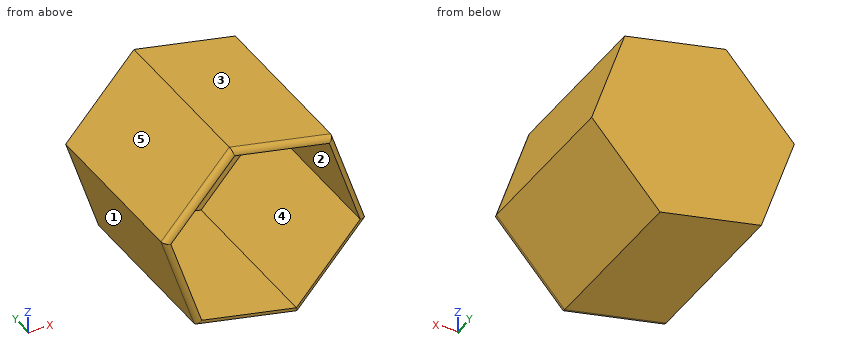
```python
from build123d import *

# Parameters (mm, degrees)
F1_DEPTH = 30
F2_T     = -1
F3_R     = 0.99999


# Not quite as in the source:
# - a fillet or chamfer is up to 0.001 mm smaller than in the source, because OpenCascade refuses the exact size


with BuildPart() as f1:
    # F0 (on Front) → F1 (new body)
    with BuildSketch(Plane.XZ):
        Polygon((-16.0683598468, 10.3036999003), (-4.4305566599, 23.5195108458), (-10.0568830769, 40.2060495226), (-27.3210126808, 43.676777254), (-38.9588158677, 30.4609663085), (-33.3324894507, 13.7744276316), align=None)
    extrude(amount=F1_DEPTH)

    # F2
    f2_openings = [f1.faces().sort_by_distance(p)[0] for p in [
        (-21.694686, -30, 26.990239),
    ]]
    offset(amount=F2_T, openings=f2_openings)

    # F3 (radius 1 in the source; OpenCascade refuses exactly that, so slightly less here)
    f3_edges = [f1.edges().sort_by_distance(p)[0] for p in [
        (-18.688948, -30, 41.941413),
        (-7.24372, -30, 31.86278),
        (-10.249458, -30, 16.911605),
        (-24.700425, -30, 12.039064),
        (-36.145653, -30, 22.117697),
        (-33.139914, -30, 37.068872),
    ]]
    fillet(f3_edges, radius=F3_R)


solid = f1.part
```
Check sheet for the modelled part. Datum: model origin and axes. Units: mm. Face numbers are marked on the shaded views. A direction names the side the tool comes from. Round coordinates to 2 decimals unless told otherwise and drop trailing zeros. Loops run counter-clockwise (first coordinate to the right, second up) from the corner with the lowest first, then second, coordinate; pieces in that order, holes last. Notation, with made-up numbers: (77.5, 17.25) -> (108.5, 17.25) arc R22 cw to (108.5, 51.25) -> close; hole circle Ø11 at (80, 84). An arc over 180 degrees is marked (long way). Write item = value, one per line. Start each with the question number.
1) Release check for a two-part mould opening along X. For the marked faces 3, 4 and 5 record: released by +X, released by -X, zero draft, split by the parting line, or undercut.
2) Thickness scan on probe 1 along Y at (x, z) = (-23, 22.5); probe 2 along Z at (x, y) = (-30.5, -23.5) (3 decimals); probe 3 along X at (y, z) = (-7, 25.5). Record the ranges inside material, lowest first.
3) Set-up check for the marked faces 1 and 2: record each of +Z, -Z, +X, -X, +Y, -Y from which the full face is reachable in a straight line by a thin tool's end or side.
4) Gauge pin test, flat ends, axial feed: pin 1 Ø3 at (y, z) = (-3, 16.5) entering from -X; pin 2 Ø12 at (x, y) = (-32, -24.5) entering from -Z; pin 3 Ø12 at (y, z) = (-6, 32.5) entering from +X. Record the tip position at first contact, or that the pin passes through.
5) Sectioned sample at A-A, the plane y = -21.5. Record the cut outline in (x, z).
Results are:
q1.face_3 = released by +X
q1.face_4 = undercut
q1.face_5 = released by -X
q2.probe_1 = -1 to 0
q2.probe_2 = 13.205 to 14.225, 38.554 to 40.067
q2.probe_3 = -37.29 to -36.23, -6.15 to -5.1
q3.face_1 = -Z, -X, +Y, -Y
q3.face_2 = -Y
q4.pin_1 = -34.76
q4.pin_2 = 12.3
q4.pin_3 = -5.44
q5.outline = (-38.96, 30.46) -> (-33.33, 13.77) -> (-16.07, 10.3) -> (-4.43, 23.52) -> (-10.06, 40.21) -> (-27.32, 43.68) -> close; hole (-37.83, 30.23) -> (-32.57, 14.64) -> (-16.44, 11.4) -> (-5.56, 23.75) -> (-10.82, 39.34) -> (-26.95, 42.58) -> close
